```python
from build123d import *

# Parameters (mm, degrees)
SKETCH1_R           = 9.25
BOSS_EXTRUDE1_DEPTH = 6.78
SKETCH2_R           = 2.05
CUT_EXTRUDE1_DEPTH  = 15.734089724
SKETCH3_R           = 3.45
CUT_EXTRUDE2_DEPTH  = 3.5
SKETCH4_R           = 1.6
CUT_EXTRUDE3_DEPTH  = 15.734089724
CIRPATTERN1_COUNT   = 2
SKETCH5_R           = 2.75
CUT_EXTRUDE4_DEPTH  = 3
CIRPATTERN2_COUNT   = 2


with BuildPart() as part:
    # Sketch1 → Boss-Extrude1 (new body)
    with BuildSketch(Plane(origin=(0, 0, 0), x_dir=(1, 0, 0), z_dir=(0, 1, 0))):
        with Locations(Location((0, 0, 0), (0, 0, 270))):
            Circle(SKETCH1_R)
    extrude(amount=BOSS_EXTRUDE1_DEPTH)

    # Sketch2 → Cut-Extrude1 (cut, through all)
    with BuildSketch(Plane(origin=(0, 6.78, 0), x_dir=(1, 0, 0), z_dir=(0, 1, 0))):
        with Locations(Location((0, 0, 0), (0, 0, 270))):
            Circle(SKETCH2_R)
    extrude(amount=-CUT_EXTRUDE1_DEPTH, mode=Mode.SUBTRACT)

    # Sketch3 → Cut-Extrude2 (cut)
    with BuildSketch(Plane(origin=(0, 6.78, 0), x_dir=(1, 0, 0), z_dir=(0, 1, 0))):
        with Locations(Location((0, 0, 0), (0, 0, 270))):
            Circle(SKETCH3_R)
    extrude(amount=-CUT_EXTRUDE2_DEPTH, mode=Mode.SUBTRACT)

    # Sketch4 → Cut-Extrude3 (cut, through all)
    with BuildSketch(Plane(origin=(0, 0, 0), x_dir=(-1, 0, 0), z_dir=(0, -1, 0))):
        with Locations(Location((0, 5.45, 0), (0, 0, 90))):
            Circle(SKETCH4_R)
    cut_extrude3 = extrude(amount=-CUT_EXTRUDE3_DEPTH, mode=Mode.SUBTRACT)

    # CirPattern1: Cut-Extrude3 ×2 about axis
    cirpattern1_axis = Axis((0, 0, 0), (0, 1, 0))
    for i in range(1, CIRPATTERN1_COUNT):
        add(cut_extrude3.rotate(cirpattern1_axis, i * 360 / CIRPATTERN1_COUNT), mode=Mode.SUBTRACT)

    # Sketch5 → Cut-Extrude4 (cut)
    with BuildSketch(Plane(origin=(0, 0, 0), x_dir=(-1, 0, 0), z_dir=(0, -1, 0))):
        with Locations(Location((0, 5.45, 0), (0, 0, 90))):
            Circle(SKETCH5_R)
    cut_extrude4 = extrude(amount=-CUT_EXTRUDE4_DEPTH, mode=Mode.SUBTRACT)

    # CirPattern2: Cut-Extrude4 ×2 about axis
    cirpattern2_axis = Axis((0, 0, 0), (0, 1, 0))
    for i in range(1, CIRPATTERN2_COUNT):
        add(cut_extrude4.rotate(cirpattern2_axis, i * 360 / CIRPATTERN2_COUNT), mode=Mode.SUBTRACT)


solid = part.part
```
Verification items for the finished model (mm, model axes). A direction names the side the tool comes from. Round coordinates to 2 decimals unless told otherwise and drop trailing zeros. Order: outer loops, then holes, each group sorted by start corner. A loop starts at its lowest first (then second) coordinate and runs counter-clockwise, first axis right, second up.
1) Depth check by flat-ended pin: pin 1 (7.5 mm diameter, centred on x = -1.5, z = -1, fed in from +Y); pin 2 (3.5 mm diameter, centred on x = 0, z = -5.45, fed in from -Y); pin 3 (4 mm diameter, centred on y = 2, z = -3, fed in from +X); pin 4 (1.5 mm diameter, centred on y = 6, z = -5, fed in from +X). Enter the tip coordinate at first touch or a pass-through.
Geometry says:
pin 1: stops at y = 6.78
pin 2: stops at y = 3
pin 3: stops at x = 9.2
pin 4: stops at x = 8.22
2) Cross-section at C-C, the plane y = 5.5. Record the cut outline in (x, z), plus the area to 3 significant figures.
Geometry says:
outline: circle Ø18.5 at (0, 0); hole circle Ø6.9 at (0, 0); hole circle Ø3.2 at (0, -5.45); hole circle Ø3.2 at (0, 5.45)
area: 215 mm2
3) Cross-section at B-B, the plane z = 0. Record the cut outline in (x, y).
Geometry says:
outline: (-9.25, 0) - (-2.05, 0) - (-2.05, 3.28) - (-3.45, 3.28) - (-3.45, 6.78) - (-9.25, 6.78) - close; (2.05, 0) - (9.25, 0) - (9.25, 6.78) - (3.45, 6.78) - (3.45, 3.28) - (2.05, 3.28) - close
4) Cross-section at A-A, the plane x = 0. Record the cut outline in (y, z).
Geometry says:
outline: (0, -9.25) - (6.78, -9.25) - (6.78, -7.05) - (3, -7.05) - (3, -8.2) - (0, -8.2) - close; (0, -2.7) - (3, -2.7) - (3, -3.85) - (6.78, -3.85) - (6.78, -3.45) - (3.28, -3.45) - (3.28, -2.05) - (0, -2.05) - close; (0, 2.05) - (3.28, 2.05) - (3.28, 3.45) - (6.78, 3.45) - (6.78, 3.85) - (3, 3.85) - (3, 2.7) - (0, 2.7) - close; (0, 8.2) - (3, 8.2) - (3, 7.05) - (6.78, 7.05) - (6.78, 9.25) - (0, 9.25) - close
5) Draft check along Z on faces 4 (the cylindrical face through (-3.543, 3.343, 8.545)), 5 (the cylindrical face through (0.481, 4.864, -6.976)), 6 (the flat face through (0.1, 0, -2.2)), 7 (the cylindrical face through (2.332, 5.054, -2.543)). Enter one of: +Z half, -Z half, draft (parallel to the pull), parting line (faces both ways), or undercut.
Geometry says:
face 4: parting line
face 5: undercut
face 6: draft
face 7: undercut
6) Cross-section at D-D, the plane z = -5.45. Record the cut outline in (x, y).
Geometry says:
outline: (-7.47, 0) - (-2.75, 0) - (-2.75, 3) - (-1.6, 3) - (-1.6, 6.78) - (-7.47, 6.78) - close; (1.6, 3) - (2.75, 3) - (2.75, 0) - (7.47, 0) - (7.47, 6.78) - (1.6, 6.78) - close
7) Tool access check on faces 1 (the cylindrical face through (-2.685, 1.479, -4.854)), 2 (the cylindrical face through (0.61, 4.86, 6.93)), 3 (the flat face through (-2.3, 3.28, 0)). Record the directions out of +Z, -Z, +X, -X, +Y, -Y that give a thin tool (end or side, any length) a straight path to the whole face; none if there is none.
Geometry says:
face 1: -Y
face 2: +Y, -Y
face 3: +Y
8) Material ranges on line 1 (X direction, y = 4.3, z = 0); line 2 (X direction, y = 1.25, z = 0); line 3 (Y direction, x = -0.5, z = -3), recorded low to high.
Geometry says:
line 1: x = -9.25 to -3.45, 3.45 to 9.25
line 2: x = -9.25 to -2.05, 2.05 to 9.25
line 3: y = 3 to 3.28
